For this review, take the finished solid that the model builds, in its own axes (mm). A direction names the side the tool comes from. Coordinates: 2 decimals unless noted, no trailing zeros. Loops run counter-clockwise (first coordinate to the right, second up) from the corner with the lowest first, then second, coordinate; pieces in that order, holes last. Notation, with made-up numbers: M 19.5,-20.75 L 56.5,-20.75 A36 cw 56.5,14.25 Z; hole C 89.5,70 d8. An arc over 180 degrees is marked long. Put each result on its own line as item: value.
```python
from build123d import *

# Parameters (mm, degrees)
SKETCH2_R          = 4.7625
CUT_EXTRUDE1_DEPTH = 34.995099077


with BuildPart() as part:
    # Sketch1 → Revolve1 (revolve)
    with BuildSketch(Plane.XY):
        Polygon((0, 0), (2.71145, 2.71145), (5.51815, -0.09525), (8.45185, 2.83845), (11.0998, 0.1905), (11.0998, -12.65555), (0, -12.65555), align=None)
    revolve(axis=Axis((11.0998, -12.65555, 0), (-1, 0, 0)))

    # Sketch2 → Cut-Extrude1 (cut, through all)
    with BuildSketch(Plane(origin=(11.0998, 0, 0), x_dir=(0, 0, -1), z_dir=(1, 0, 0))):
        with Locations(Location((0, -12.65555, 0), (0, 0, 90))):
            Circle(SKETCH2_R)
    extrude(amount=-CUT_EXTRUDE1_DEPTH, mode=Mode.SUBTRACT)


solid = part.part
```
(1) Wall thickness on line 1 along Z through (x, y) = (5.5, -12.5); line 2 along Z through (x, y) = (4, -6.5); line 3 along Y through (x, z) = (7.5, -3.5): over which ranges is each line inside the solid? List them lowest first. Write a range as [from, to].
Determined:
line 1: z = [-12.58, -4.76], [4.76, 12.58]
line 2: z = [-12.66, 12.66]
line 3: y = [-26.77, -15.89], [-9.43, 1.46]
(2) Add section C-C (x = 10). Write out the cut boundary in (y, z) (1 decimal), plus the area to 3 significant figures.
Determined:
outline: C -12.7,0 d27.9; hole C -12.7,0 d9.5
area: 540 mm^2
(3) Tool access review of faces 4 (the conical face through (10.97, -25.62, -0.57)), 5 (the conical face through (5.7, -15.42, 12.44)): name each direction out of +Z, -Z, +X, -X, +Y, -Y from which nothing blocks a thin tool from reaching the whole face with its end or side.
Determined:
face 4: +X
face 5: none
(4) For pin 1 (1 mm diameter, centred on x = 7, z = -10, fed in from -Y); pin 2 (15 mm diameter, centred on y = -12.66, z = 0, fed in from +X); pin 3 (3 mm diameter, centred on x = 7.5, z = -3, fed in from +Y); pin 4 (2 mm diameter, centred on x = 1.5, z = -4, fed in from -Y), all flat-tipped, find the tip position at first contact; note any pin that passes through.
Determined:
pin 1: stops at y = -23.36
pin 2: stops at x = 11.1
pin 3: stops at y = 2.73
pin 4: stops at y = -27.31
(5) Draft analysis for pull direction Z (two halves, no side actions). For faces 1 (the flat face through (0, -12, 5)), 2 (the conical face through (0.17, -15.44, 12.52)), 3 (the cylindrical face through (5.628, -17.413, 0.209)), state which applies: +Z half, -Z half, draft (parallel to the pull), parting line (faces both ways), or undercut.
Determined:
face 1: draft
face 2: parting line
face 3: undercut
(6) Add section A-A (z = 0). Write out the cut boundary in (x, y), plus the area to 3 significant figures.
Determined:
outline: M 0,-25.31 L 2.71,-28.02 L 5.52,-25.22 L 8.45,-28.15 L 11.1,-25.5 L 11.1,-17.42 L 0,-17.42 Z; M 0,-7.89 L 11.1,-7.89 L 11.1,0.19 L 8.45,2.84 L 5.52,-0.1 L 2.71,2.71 L 0,0 Z
area: 206 mm^2
